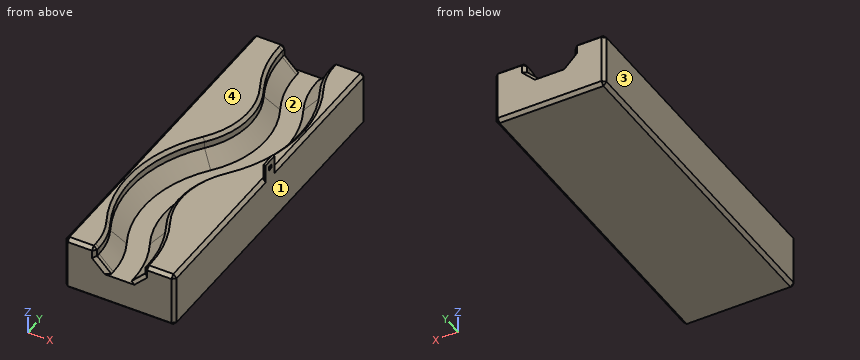
from build123d import *

# Parameters (mm, degrees)
SKETCH1_W                = 50
SKETCH1_H                = 150
BOSS_EXTRUDE1_DEPTH      = 25
CHAMFER1_SIZE            = 1.5
BOSS_EXTRUDE2_DEPTH      = 7
BOSS_EXTRUDE2_DEPTH_BACK = 10
SKETCH4_W                = 1
SKETCH4_H                = 7
SKETCH5_W                = 1.8
SKETCH5_H                = 1.8
CUT_EXTRUDE1_DEPTH       = 7


with BuildPart() as part:
    # Sketch1 → Boss-Extrude1 (new body)
    with BuildSketch(Plane.XY):
        with Locations((25, 75)):
            Rectangle(SKETCH1_W, SKETCH1_H)
    extrude(amount=BOSS_EXTRUDE1_DEPTH)

    # Cut-Sweep1: sweep along a path in Sketch3
    with BuildLine(Plane.XY.offset(25)) as cut_sweep1_path:
        Line((25, 0), (25, 3))
        ThreePointArc((25, 3), (23.751063127, 13.408967361), (20.075154476, 23.227019124))
        ThreePointArc((20.075154476, 23.227019124), (14.918298123, 49.838284764), (25, 75))
        ThreePointArc((25, 75), (35.081701877, 100.161715236), (29.924845524, 126.772980876))
        ThreePointArc((29.924845524, 126.772980876), (26.248936873, 136.591032639), (25, 147))
        Line((25, 147), (25, 150))
    # Sketch2 → Cut-Sweep1 (sweep, cut)
    with BuildSketch(Plane.XZ):
        Polygon((29.556349186, 36), (20.443650814, 36), (14, 29.556349186), (14, 20.443650814), (20.443650814, 14), (29.556349186, 14), (36, 20.443650814), (36, 29.556349186), align=None)
    sweep(path=cut_sweep1_path.line, mode=Mode.SUBTRACT)

    # Chamfer1
    chamfer1_edges = [part.edges().sort_by_distance(p)[0] for p in [
        (50, 75, 25),
        (43, 150, 25),
        (43, 0, 25),
        (7, 150, 25),
        (14, 1.5, 25),
        (13.063297345, 10.806725521, 25),
        (3.967729924, 50.879945025, 25),
        (24.131133677, 101.203375498, 25),
        (15.561171091, 133.988790799, 25),
        (14, 148.5, 25),
        (36, 1.5, 25),
        (34.438828909, 16.011209201, 25),
        (25.868866323, 48.796624502, 25),
        (46.032270076, 99.120054975, 25),
        (36.936702655, 139.193274479, 25),
        (36, 148.5, 25),
        (36, 150, 22.721825407),
        (14, 150, 22.721825407),
        (36, 0, 22.721825407),
        (14, 0, 22.721825407),
        (17.221825407, 0, 17.221825407),
        (32.778174593, 0, 17.221825407),
        (32.778174593, 150, 17.221825407),
        (17.221825407, 150, 17.221825407),
        (0, 75, 25),
        (25, 150, 0),
        (50, 75, 0),
        (25, 0, 0),
        (0, 75, 0),
        (7, 0, 25),
        (0, 150, 12.5),
        (50, 150, 12.5),
        (50, 0, 12.5),
        (0, 0, 12.5),
    ]]
    chamfer(chamfer1_edges, length=CHAMFER1_SIZE)

    # Sketch4 → Boss-Extrude2 (add, two sides: drawn at the far end of the back side and taken through both)
    with BuildSketch(Plane.XY.offset(25).offset(-BOSS_EXTRUDE2_DEPTH_BACK)):
        with Locations((49.5, 75)):
            Rectangle(SKETCH4_W, SKETCH4_H)
    extrude(amount=BOSS_EXTRUDE2_DEPTH + BOSS_EXTRUDE2_DEPTH_BACK)

    # Sketch5 → Cut-Extrude1 (cut)
    with BuildSketch(Plane(origin=(50, 0, 0), x_dir=(0, 0, -1), z_dir=(1, 0, 0))):
        with Locations((-28.6, 75)):
            Rectangle(SKETCH5_W, SKETCH5_H)
    extrude(amount=-CUT_EXTRUDE1_DEPTH, mode=Mode.SUBTRACT)


solid = part.part
Geometry: final body of the model. Coordinates: model frame, mm. Face numbers are marked on the shaded views. Coordinates: 2 decimals unless noted, no trailing zeros. Order: outer loops, then holes, each group sorted by start corner. A loop starts at its lowest first (then second) coordinate and runs counter-clockwise, first axis right, second up.
1) Draft query along X for the marked faces 1, 2, 3 and 4. Return one class per face: released by +X, released by -X, zero draft, split by the parting line, or undercut.
Result sheet:
face 1: released by +X
face 2: undercut
face 3: released by -X
face 4: zero draft
2) Section A-A (z = 18.5). Return loops of the section in (x, y).
Result sheet:
outline: (0, 1.5) - (1.5, 0) - (13.82, 0) - (15.94, 1.5) - (15.94, 3) arc R34.94 ccw to (12.03, 19.06) arc R57.06 cw to (17.89, 80.6) arc R38.94 ccw to (21.88, 122.61) arc R53.06 cw to (15.94, 147) - (15.94, 148.5) - (13.82, 150) - (1.5, 150) - (0, 148.5) - close; (28.12, 27.39) arc R53.06 cw to (34.06, 3) - (34.06, 1.5) - (36.18, 0) - (48.5, 0) - (50, 1.5) - (50, 148.5) - (48.5, 150) - (36.18, 150) - (34.06, 148.5) - (34.06, 147) arc R34.94 ccw to (37.97, 130.94) arc R57.06 cw to (32.11, 69.4) arc R38.94 ccw to start
3) First-contact query: P1, Ø0.5, axis at x = 49.5, z = 28.5, coming from the +Y side; P2, Ø5.5, axis at y = 76.5, z = 27.5, coming from the -X side; P3, Ø23.5, axis at x = 32.5, y = 76.5, coming from the +Z side. Flat tips, straight axial feed; report the tip coordinate or a pass-through.
Result sheet:
P1: stops at y = 78.5
P2: stops at x = 1.25
P3: stops at z = 25
4) Ray query, probe 1 along X at (y, z) = (29.5, 17.5); probe 2 along Z at (x, y) = (33, 118); probe 3 along X at (y, z) = (44, 18). Return the intervals inside material, ascending.
Result sheet:
probe 1: x = 0 to 8.92, 26.01 to 50
probe 2: z = 0 to 14
probe 3: x = 0 to 6.16, 23.28 to 50
